Autodesk Inventor part; units mm, degrees
ref_plane "MSC_PF1" through (0, 0, 0) normal (0, 1, 0) x (-1, 0, 0)
ref_plane "MSC_PT1" through (0, 0, 18.7798) normal (0, 0, -1) x (-1, 0, 0)
ref_plane "YZ Plane" through (0, 0, 0) normal (1, 0, 0) x (0, 1, 0)
sketch "Schizzo2" plane through (0, 0, 0) normal (0, 1, 0) x (-1, 0, 0)
  line L0 (0, 18.7798) -> (0, -36.2202)
  line L1 (0, -36.2202) -> (7, -36.2202)
  line L2 (8, -35.2202) -> (8, 1.7798)
  line L3 (8, 1.7798) -> (7.25, 3.0788)
  line L4 (7.25, 3.0788) -> (7.25, 18.7798)
  line L5 (7.25, 18.7798) -> (0, 18.7798)
  line L6 (7, -36.2202) -> (8, -35.2202)
  line L7 (8, -36.2202) -> (8, -37.6344)
  line L8 (0, -48.9172) -> (0, 30.0627)
  dimension "Ds" = 14.5
  dimension "NND" = 16
  dimension "b" = 38
  dimension "d3" = 30
  dimension "d5" = 45
  dimension "PTC" = 2
  dimension "NLG" = 55
revolve "Rivoluzione1" add sketch "Schizzo2" angle 360 about axis through (0, 0, 18.7798) along (0, 0, -1)
sketch "Schizzo3" plane through (0, 0, 18.7798) normal (0, 0, 1) x (1, 0, 0)
  circle A0 centre (0, 0) radius 7.25
  line L0 (0, 12) -> (6.9282, 12)
  line L1 (6.9282, 12) -> (13.8564, 0)
  line L2 (13.8564, 0) -> (0, 0)
  line L3 (0, 0) -> (0, 12)
  line L4 (0, 12) -> (-6.9282, 12)
  line L5 (-6.9282, 12) -> (-13.8564, 0)
  line L6 (0, -12) -> (6.9282, -12)
  line L7 (6.9282, -12) -> (13.8564, 0)
  line L8 (-6.9282, -12) -> (-13.8564, 0)
  line L9 (0, -12) -> (-6.9282, -12)
  dimension "d9" = 60
  dimension "ParS" = 24
  dimension "msp_d11" = 24
extrude "Estrusione1" add sketch "Schizzo3" along normal blind 10
sketch "Schizzo4" plane through (0, 0, 0) normal (0, 1, 0) x (-1, 0, 0)
  line L0 (-12, 28.7798) -> (-13.8564, 28.7798)
  line L1 (-13.8564, 28.7798) -> (-13.8564, 27.708)
  line L2 (-13.8564, 27.708) -> (-12, 28.7798)
  line L3 (0, 16.7798) -> (0, 30.7798)
  line L4 (0, 28.2505) -> (0, 27.1787)
  line L5 (-13.8564, 18.7798) -> (-13.8564, 28.7798)
  line L6 (-6.9282, 28.7798) -> (-13.8564, 28.7798)
  dimension "d14" = 30
  dimension "msp_d15" = 24
revolve "Rivoluzione2" cut sketch "Schizzo4" angle 360 about axis through (0, 0, 28.2505) along (0, 0, -1)
sketch "Sketch5" plane through (0, 0, 28.7798) normal (0, 0, 1) x (1, 0, 0)
  arc A0 (10.3923, 6) -> (0, 12) centre (0, 0) ccw
  circle A1 centre (0, 0) radius 9
  dimension "d27" = 18
extrude "Extrusion2" cut sketch "Sketch5" against normal blind 2
thread "Filettatura1"
ref_plane "MSC_PF1" through (0, 0, 0) normal (0, 1, 0) x (-1, 0, 0)
ref_plane "MSC_PT1" through (0, 0, 18.7798) normal (0, 0, -1) x (-1, 0, 0)
fillet "Fillet1" radius 0.6 1 edges at (7.25, 0, 18.7798)
equation "\"d27\" = 0.75 * ParS"
equation "\"d28\" = 0.2 * ParK"
equation "\"d30\" = r"
equation "\"msp_d11\" = ParS"
equation "\"msp_d17\" = b"
equation "\"msp_d15\" = ParS"
equation "\"r\" = 0.6"
equation "\"THREADDIA\" = NND"
properties part number "BS EN ISO 4015 - M16x55" material "Acciaio inox, 440C"
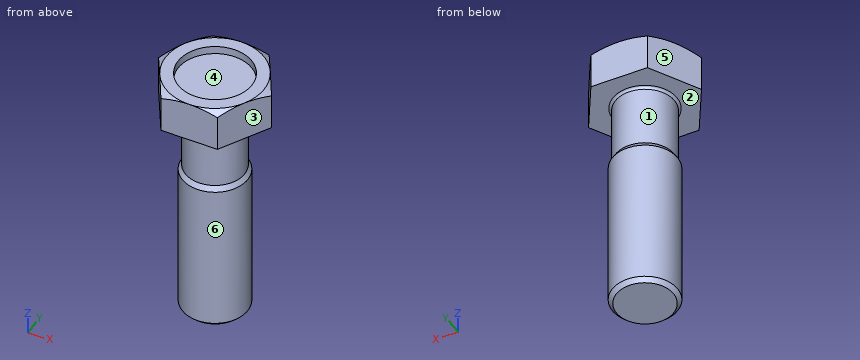
CAD build for the part. Positions are in the model's coordinates, mm. Face numbers are marked on the shaded views. A direction names the side the tool comes from. Round coordinates to 2 decimals unless told otherwise and drop trailing zeros. Loops run counter-clockwise (first coordinate to the right, second up) from the corner with the lowest first, then second, coordinate; pieces in that order, holes last.
(1) Wall check: line 1 along Y through (x, z) = (0, 27.3); line 2 along Z through (x, y) = (8, 5.75); line 3 along Z through (x, y) = (-5.5, 3.25). Give the ranges that are in metal, low to high.
(2) Two-plate mould, pull along X, no slides. Class the marked faces 1, 2, 3 and 4: +X half, -X half, draft (parallel to the pull), parting line (faces both ways), or undercut.
(3) Cut at A-A (z = -9.5). Give the cut face in (x, y).
(4) Cut at B-B (z = 22). Give the cut face in (x, y), plus the area to 3 significant figures.
(5) Drop flat-ended pins along their axis: pin 1 (4 mm diameter, centred on x = -0.5, y = 3.5, fed in from +Z); pin 2 (10 mm diameter, centred on x = 4.5, y = -7, fed in from -Z); pin 3 (8 mm diameter, centred on x = -11, z = -22, fed in from +Y); pin 4 (4 mm diameter, centred on y = -6, z = -18.5, fed in from +X). Give the stop position or say it passes through.
(6) Which spindle directions (+Z, -Z, +X, -X, +Y, -Y) get a long thin tool onto all of the face, cutting with end or side? Do the marked faces 5 and 6. Say none if no direction does.
(7) Cut at C-C (z = 4). Give the cut face in (x, y), plus the area to 3 significant figures.
Findings below:
1. line 1: y = -12 to -9, 9 to 12
1. line 2: z = 18.78 to 28.78
1. line 3: z = -36.22 to 26.78
2. face 1: parting line
2. face 2: draft
2. face 3: +X half
2. face 4: undercut
3. outline: circle Ø16 at (0, 0)
4. outline: (-13.86, 0) - (-6.93, -12) - (6.93, -12) - (13.86, 0) - (6.93, 12) - (-6.93, 12) - close
4. area: 499 mm2
5. pin 1: stops at z = 26.78
5. pin 2: stops at z = -36.22
5. pin 3: stops at y = 3.87
5. pin 4: stops at x = 6.93
6. face 5: +Z, -Z, -X, +Y
6. face 6: -Z
7. outline: circle Ø14.5 at (0, 0)
7. area: 165 mm2
